Geometry check sheet. Reference: the model listing, model coordinates, mm. A direction names the side the tool comes from. Coordinates: 2 decimals unless noted, no trailing zeros. Loops run counter-clockwise (first coordinate to the right, second up) from the corner with the lowest first, then second, coordinate; pieces in that order, holes last. Notation, with made-up numbers: (-8.5, 64) - (47.5, 64) arc R12 cw to (47.5, 78) - close; hole circle Ø5 at (82.5, 71). An arc over 180 degrees is marked (long way). Write item = value, one per line. Start each with the question number.
from build123d import *

# Parameters (mm, degrees)
SKETCH1_R           = 31.75
BOSS_EXTRUDE1_DEPTH = 1.5875
SKETCH3_W           = 50.8
SKETCH3_H           = 41.275
CUT_EXTRUDE1_DEPTH  = 1.5875
CUT_EXTRUDE2_REACH  = 3.587
SKETCH4_W           = 38.1
SKETCH4_H           = 25.4
FILLET3_R           = 2.54


with BuildPart() as part:
    # Sketch1 → Boss-Extrude1 (new body, symmetric)
    with BuildSketch(Plane.XY):
        Circle(SKETCH1_R)
    extrude(amount=BOSS_EXTRUDE1_DEPTH, both=True)

    # Sketch3 → Cut-Extrude1 (cut)
    with BuildSketch(Plane(origin=(0, 0, -1.5875), x_dir=(-1, 0, 0), z_dir=(0, 0, -1))):
        Rectangle(SKETCH3_W, SKETCH3_H)
    extrude(amount=-CUT_EXTRUDE1_DEPTH, mode=Mode.SUBTRACT)

    # Sketch4 → Cut-Extrude2 (cut, up to next)
    with BuildSketch(Plane(origin=(0, 0, 0), x_dir=(-1, 0, 0), z_dir=(0, 0, -1)), mode=Mode.PRIVATE) as cut_extrude2_sk1:
        Rectangle(SKETCH4_W, SKETCH4_H)
    cut_extrude2_tool1 = extrude(cut_extrude2_sk1.sketch, amount=-CUT_EXTRUDE2_REACH, mode=Mode.PRIVATE) & part.part
    add(cut_extrude2_tool1.solids().sort_by_distance((0, 0, 0))[0], mode=Mode.SUBTRACT)

    # Fillet3
    fillet3_edges = [part.edges().sort_by_distance(p)[0] for p in [
        (-19.05, 12.7, 0.79375),
        (-19.05, -12.7, 0.79375),
        (19.05, -12.7, 0.79375),
        (19.05, 12.7, 0.79375),
    ]]
    fillet(fillet3_edges, radius=FILLET3_R)


solid = part.part
(1) Scan lines: line 1 (Z direction, x = -4, y = -20); line 2 (Y direction, x = -16, z = 1.2); line 3 (Y direction, x = -6, z = 0.65). Record each from-to range of solid material in increasing order.
(2) Draft check along Y on faces 5 (the face through (19.05, 0, 1)), 6 (the face through (28, 0, -1.588)), 7 (the face through (30.284, 9.537, 0.022)). Enter one of: pulls with the +Y half, pulls with the -Y half, needs draft (parallel to the pull), parting line crosses it, or undercut.
(3) Sectioned sample at B-B on x = 9. Enter the section's corners in (y, z), plus the area to 3 significant figures.
(4) Sectioned sample at C-C on x = 22.5. Enter the section's corners in (y, z).
(5) Sectioned sample at D-D on y = 15. Enter the section's corners in (x, z), plus the area to 3 significant figures.
(6) Depth check by flat-ended pin: pin 1 (1.3 mm diameter, centred on y = -4.5, z = 0.5, fed in from -X); pin 2 (1.3 mm diameter, centred on x = -10.5, z = -1, fed in from -Y); pin 3 (10 mm diameter, centred on x = 23, y = 3.5, fed in from -Z); pin 4 (1 mm diameter, centred on x = -4.5, z = 0, fed in from -Y). Enter the tip coordinate at first touch or a pass-through.
(7) Sectioned sample at A-A on y = -5.5. Enter the section's corners in (x, z), plus the area to 3 significant figures.
(8) Tool access check on faces 1 (the face through (18.326, 11.936, 0.805)), 2 (the face through (25.4, 0, -1)), 3 (the face through (0, -20.638, -1)), 4 (the face through (0, 14, 0)). Record the directions out of +Z, -Z, +X, -X, +Y, -Y that give a thin tool (end or side, any length) a straight path to the whole face; none if there is none.
Working result:
q1.line_1 = 0 to 1.59
q1.line_2 = -27.42 to -12.7, 12.7 to 27.42
q1.line_3 = -31.18 to -12.7, 12.7 to 31.18
q2.face_5 = undercut
q2.face_6 = needs draft
q2.face_7 = parting line crosses it
q3.outline = (-30.45, -1.59) - (-20.64, -1.59) - (-20.64, 0) - (-12.7, 0) - (-12.7, 1.59) - (-30.45, 1.59) - close; (12.7, 0) - (20.64, 0) - (20.64, -1.59) - (30.45, -1.59) - (30.45, 1.59) - (12.7, 1.59) - close
q3.area = 87.5 mm2
q4.outline = (-22.4, -1.59) - (-20.64, -1.59) - (-20.64, 0) - (20.64, 0) - (20.64, -1.59) - (22.4, -1.59) - (22.4, 1.59) - (-22.4, 1.59) - close
q5.outline = (-27.98, -1.59) - (-25.4, -1.59) - (-25.4, 0) - (25.4, 0) - (25.4, -1.59) - (27.98, -1.59) - (27.98, 1.59) - (-27.98, 1.59) - close
q5.area = 97.0 mm2
q6.pin_1 = -31.52
q6.pin_2 = -30.18
q6.pin_3 = -1.59
q6.pin_4 = -31.5
q7.outline = (-31.27, -1.59) - (-25.4, -1.59) - (-25.4, 0) - (-19.05, 0) - (-19.05, 1.59) - (-31.27, 1.59) - close; (19.05, 0) - (25.4, 0) - (25.4, -1.59) - (31.27, -1.59) - (31.27, 1.59) - (19.05, 1.59) - close
q7.area = 57.4 mm2
q8.face_1 = +Z, -Z
q8.face_2 = -Z, +Y, -Y
q8.face_3 = -Z, +X, -X
q8.face_4 = -Z
